Here's how the part is built. I have some questions about the finished solid (model axes, mm). Face numbers are marked on the shaded views. A direction names the side the tool comes from. Give positions to 0.01 mm unless a question says otherwise; leave off trailing zeros. Loops run counter-clockwise (first coordinate to the right, second up) from the corner with the lowest first, then second, coordinate; pieces in that order, holes last.
Q1. I'm going to push flat-ended pins straight in: P1, Ø1.5, axis at x = 35, y = -3, coming from the +Z side; P2, Ø4, axis at x = 19.5, z = 21, coming from the +Y side; P3, Ø5, axis at x = 10, y = -10, coming from the +Z side. Where does each tip first touch, or does it pass through?
Q2. I need wall thicknesses on probe 1 along Y at (x, z) = (45, 2.3); probe 2 along X at (y, z) = (-39.5, 42.5); probe 3 along Y at (x, z) = (27, 1). Which ranges of each line are inside material? Lowest first, please.
Q3. Suppose I cut it at A-A (z = 44). List the corners of the cut face in (x, y) for me, and give its area (3 significant figures).
Q4. For the marked faces 5 and 6, which set-ups out of +Z, -Z, +X, -X, +Y, -Y let a thin tool reach every point of the face, with its end or its side?
Q5. Suppose I cut it at C-C (y = -27.5). List the corners of the cut face in (x, z) for me.
Q6. Suppose I cut it at B-B (x = 45). List the corners of the cut face in (y, z) for me, and give its area (3 significant figures).
Q7. Thinking about a two-plate mould opening in X: for the marked faces 1, 2, 3 and 4, which applies, pulls with the +X half, pulls with the -X half, needs draft (parallel to the pull), parting line crosses it, or undercut?
Q8. Suppose I cut it at D-D (x = 27.5). List the corners of the cut face in (y, z) for me, and give its area (3 significant figures).
```python
from build123d import *

# Parameters (mm, degrees)
CROQUIS1_W              = 55
CROQUIS1_H              = 55
SALIENTE_EXTRUIR1_DEPTH = 60
CROQUIS2_W              = 45
CROQUIS2_H              = 45
CORTAR_EXTRUIR1_DEPTH   = 55
CORTAR_EXTRUIR2_REACH   = 57
CROQUIS3_W              = 18
CROQUIS3_H              = 40
CORTAR_EXTRUIR3_REACH   = 57
CROQUIS4_W              = 45
CROQUIS4_H              = 45
CORTAR_EXTRUIR4_REACH   = 62
CROQUIS5_R              = 1.5
CROQUIS5_R_2            = 15
SALIENTE_EXTRUIR2_DEPTH = 35
REDONDEO3_R             = 5
CORTAR_EXTRUIR5_REACH   = 7
CROQUIS7_W              = 5.5
CROQUIS7_H              = 30
REDONDEO4_R             = 2


with BuildPart() as part:
    # Croquis1 → Saliente-Extruir1 (new body)
    with BuildSketch(Plane.XY):
        with Locations((27.5, -27.5)):
            Rectangle(CROQUIS1_W, CROQUIS1_H)
    extrude(amount=SALIENTE_EXTRUIR1_DEPTH)

    # Croquis2 → Cortar-Extruir1 (cut)
    with BuildSketch(Plane.XY.offset(60)):
        with Locations((27.5, -27.5)):
            Rectangle(CROQUIS2_W, CROQUIS2_H)
    extrude(amount=-CORTAR_EXTRUIR1_DEPTH, mode=Mode.SUBTRACT)

    # Croquis3 → Cortar-Extruir2 (cut, up to next)
    with BuildSketch(Plane.XZ.offset(55), mode=Mode.PRIVATE) as cortar_extruir2_sk1:
        with Locations((27.5, 40)):
            Rectangle(CROQUIS3_W, CROQUIS3_H)
    cortar_extruir2_tool1 = extrude(cortar_extruir2_sk1.sketch, amount=-CORTAR_EXTRUIR2_REACH, mode=Mode.PRIVATE) & part.part
    add(cortar_extruir2_tool1.solids().sort_by_distance((27.5, -55, 40))[0], mode=Mode.SUBTRACT)

    # Croquis4 → Cortar-Extruir3 (cut, up to next)
    with BuildSketch(Plane(origin=(0, 0, 0), x_dir=(1, 0, 0), z_dir=(0, 1, 0)), mode=Mode.PRIVATE) as cortar_extruir3_sk1:
        with Locations((27.5, -37.5)):
            Rectangle(CROQUIS4_W, CROQUIS4_H)
    cortar_extruir3_tool1 = extrude(cortar_extruir3_sk1.sketch, amount=-CORTAR_EXTRUIR3_REACH, mode=Mode.PRIVATE) & part.part
    add(cortar_extruir3_tool1.solids().sort_by_distance((27.5, 0, 37.5))[0], mode=Mode.SUBTRACT)

    # Croquis5 → Cortar-Extruir4 (cut, up to next)
    with BuildSketch(Plane(origin=(0, 0, 0), x_dir=(-1, 0, 0), z_dir=(0, 0, -1)), mode=Mode.PRIVATE) as cortar_extruir4_sk1:
        with Locations((-45, -10)):
            Circle(CROQUIS5_R)
    cortar_extruir4_tool1 = extrude(cortar_extruir4_sk1.sketch, amount=-CORTAR_EXTRUIR4_REACH, mode=Mode.PRIVATE) & part.part
    add(cortar_extruir4_tool1.solids().sort_by_distance((45, -10, 0))[0], mode=Mode.SUBTRACT)
    # Croquis5 → Cortar-Extruir4 (cut, up to next)
    with BuildSketch(Plane(origin=(0, 0, 0), x_dir=(-1, 0, 0), z_dir=(0, 0, -1)), mode=Mode.PRIVATE) as cortar_extruir4_sk2:
        with Locations((-10, -10)):
            Circle(CROQUIS5_R)
    cortar_extruir4_tool2 = extrude(cortar_extruir4_sk2.sketch, amount=-CORTAR_EXTRUIR4_REACH, mode=Mode.PRIVATE) & part.part
    add(cortar_extruir4_tool2.solids().sort_by_distance((10, -10, 0))[0], mode=Mode.SUBTRACT)
    # Croquis5 → Cortar-Extruir4 (cut, up to next)
    with BuildSketch(Plane(origin=(0, 0, 0), x_dir=(-1, 0, 0), z_dir=(0, 0, -1)), mode=Mode.PRIVATE) as cortar_extruir4_sk3:
        with Locations((-45, -45)):
            Circle(CROQUIS5_R)
    cortar_extruir4_tool3 = extrude(cortar_extruir4_sk3.sketch, amount=-CORTAR_EXTRUIR4_REACH, mode=Mode.PRIVATE) & part.part
    add(cortar_extruir4_tool3.solids().sort_by_distance((45, -45, 0))[0], mode=Mode.SUBTRACT)
    # Croquis5 → Cortar-Extruir4 (cut, up to next)
    with BuildSketch(Plane(origin=(0, 0, 0), x_dir=(-1, 0, 0), z_dir=(0, 0, -1)), mode=Mode.PRIVATE) as cortar_extruir4_sk4:
        with Locations((-10, -45)):
            Circle(CROQUIS5_R)
    cortar_extruir4_tool4 = extrude(cortar_extruir4_sk4.sketch, amount=-CORTAR_EXTRUIR4_REACH, mode=Mode.PRIVATE) & part.part
    add(cortar_extruir4_tool4.solids().sort_by_distance((10, -45, 0))[0], mode=Mode.SUBTRACT)
    # Croquis5 → Cortar-Extruir4 (cut, up to next)
    with BuildSketch(Plane(origin=(0, 0, 0), x_dir=(-1, 0, 0), z_dir=(0, 0, -1)), mode=Mode.PRIVATE) as cortar_extruir4_sk5:
        with Locations((-27.5, -27.5)):
            Circle(CROQUIS5_R_2)
    cortar_extruir4_tool5 = extrude(cortar_extruir4_sk5.sketch, amount=-CORTAR_EXTRUIR4_REACH, mode=Mode.PRIVATE) & part.part
    add(cortar_extruir4_tool5.solids().sort_by_distance((27.5, -27.5, 0))[0], mode=Mode.SUBTRACT)

    # Croquis6 → Saliente-Extruir2 (add)
    with BuildSketch(Plane.XY.offset(60)):
        Polygon((50, 0), (55, 0), (55, -55), (36.5, -55), (36.5, -50), (50, -50), align=None)
    extrude(amount=SALIENTE_EXTRUIR2_DEPTH)

    # Redondeo3
    redondeo3_edges = [part.edges().sort_by_distance(p)[0] for p in [
        (36.5, -52.5, 20),
        (18.5, -52.5, 60),
        (18.5, -52.5, 20),
        (2.5, 0, 60),
        (36.5, -52.5, 95),
        (52.5, 0, 95),
    ]]
    fillet(redondeo3_edges, radius=REDONDEO3_R)

    # Croquis7 → Cortar-Extruir5 (cut, up to next)
    with BuildSketch(Plane.ZY.offset(-50), mode=Mode.PRIVATE) as cortar_extruir5_sk1:
        with Locations((87.25, -32)):
            Rectangle(CROQUIS7_W, CROQUIS7_H)
    cortar_extruir5_tool1 = extrude(cortar_extruir5_sk1.sketch, amount=-CORTAR_EXTRUIR5_REACH, mode=Mode.PRIVATE) & part.part
    add(cortar_extruir5_tool1.solids().sort_by_distance((50, -32, 87.25))[0], mode=Mode.SUBTRACT)
    # Croquis7 → Cortar-Extruir5 (cut, up to next)
    with BuildSketch(Plane.ZY.offset(-50), mode=Mode.PRIVATE) as cortar_extruir5_sk2:
        with Locations((71.75, -32)):
            Rectangle(CROQUIS7_W, CROQUIS7_H)
    cortar_extruir5_tool2 = extrude(cortar_extruir5_sk2.sketch, amount=-CORTAR_EXTRUIR5_REACH, mode=Mode.PRIVATE) & part.part
    add(cortar_extruir5_tool2.solids().sort_by_distance((50, -32, 71.75))[0], mode=Mode.SUBTRACT)

    # Redondeo4
    redondeo4_edges = [part.edges().sort_by_distance(p)[0] for p in [
        (52.5, -47, 84.5),
        (52.5, -17, 84.5),
        (52.5, -17, 90),
        (52.5, -47, 90),
        (52.5, -47, 69),
        (52.5, -17, 69),
        (52.5, -17, 74.5),
        (52.5, -47, 74.5),
    ]]
    fillet(redondeo4_edges, radius=REDONDEO4_R)


solid = part.part
```
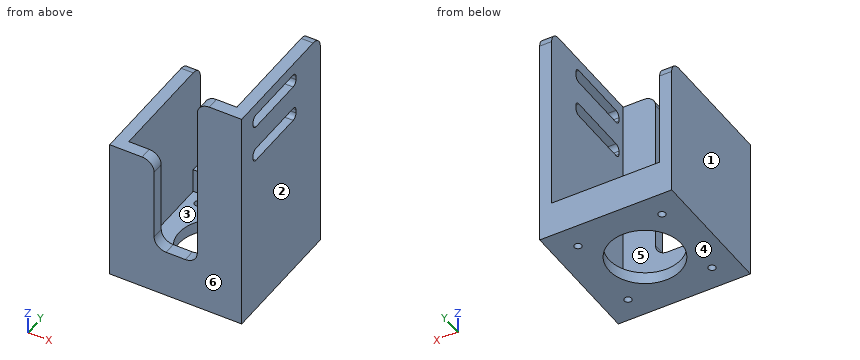
Solutions:
1. P1: stops at z = 15
1. P2: stops at y = -50
1. P3: stops at z = 5
2. probe 1: y = -55 to -46.5, -43.5 to -11.5, -8.5 to 0
2. probe 2: x = 0 to 5, 50 to 55
2. probe 3: y = -55 to -42.49, -12.51 to 0
3. outline: (0, -55) - (18.5, -55) - (18.5, -50) - (5, -50) - (5, 0) - (0, 0) - close; (36.5, -55) - (55, -55) - (55, 0) - (50, 0) - (50, -50) - (36.5, -50) - close
3. area: 685 mm2
4. face 5: +Z
4. face 6: +Z, -Z, +X, -X, -Y
5. outline: (0, 0) - (12.5, 0) - (12.5, 5) - (5, 5) - (5, 60) - (0, 60) - close; (42.5, 0) - (55, 0) - (55, 69) - (50, 69) - (50, 5) - (42.5, 5) - close; (50, 74.5) - (55, 74.5) - (55, 84.5) - (50, 84.5) - close; (50, 90) - (55, 90) - (55, 95) - (50, 95) - close
6. outline: (-55, 0) - (-46.5, 0) - (-46.5, 5) - (-50, 5) - (-50, 95) - (-55, 95) - close; (-43.5, 0) - (-11.5, 0) - (-11.5, 5) - (-43.5, 5) - close; (-8.5, 0) - (0, 0) - (0, 15) - (-5, 15) - (-5, 5) - (-8.5, 5) - close
6. area: 745 mm2
7. face 1: pulls with the -X half
7. face 2: pulls with the +X half
7. face 3: undercut
7. face 4: needs draft
8. outline: (-55, 0) - (-42.5, 0) - (-42.5, 5) - (-50, 5) - (-50, 20) - (-55, 20) - close; (-12.5, 0) - (0, 0) - (0, 15) - (-5, 15) - (-5, 5) - (-12.5, 5) - close
8. area: 250 mm2
